Autodesk Inventor part; units mm, degrees
ref_plane "Work Plane1" through (-6.65, 6.65, 6.5) normal (0, 1, 0) x (1, 0, 0)
ref_plane "YZ Plane" through (0, 0, 0) normal (1, 0, 0) x (0, 1, 0)
ref_plane "XZ Plane" through (0, 0, 0) normal (0, 1, 0) x (-1, 0, 0)
sketch "Sketch1" plane through (0, 0, 0) normal (0, 0, 1) x (1, 0, 0)
  circle A0 centre (0, 0) radius 6.65
  dimension "d0" = 13.3
extrude "Extrusion1" add sketch "Sketch1" along normal blind 6.5
ref_plane "Work Plane1" through (-6.65, 6.65, 6.5) normal (0, 1, 0) x (1, 0, 0)
sketch "Sketch3" plane through (-6.65, 6.65, 6.5) normal (0, 1, 0) x (1, 0, 0)
  circle A0 centre (6.65, 3.25) radius 1.2
  dimension "d9" = 2.4
hole "Hole1" at (0, 6.65, 3.25) direction (0, -1, 0) diameter 2.459 depth 6.65
sketch "Sketch4" plane through (0, 0, 6.5) normal (0, 0, 1) x (1, 0, 0)
  circle A0 centre (0, 0) radius 6.65
  circle A1 centre (0, 0) radius 3
  dimension "d17" = 6
extrude "Extrusion3" add sketch "Sketch4" along normal blind 4.7 contours A1
properties part number "hridel kuzelova kolecka"
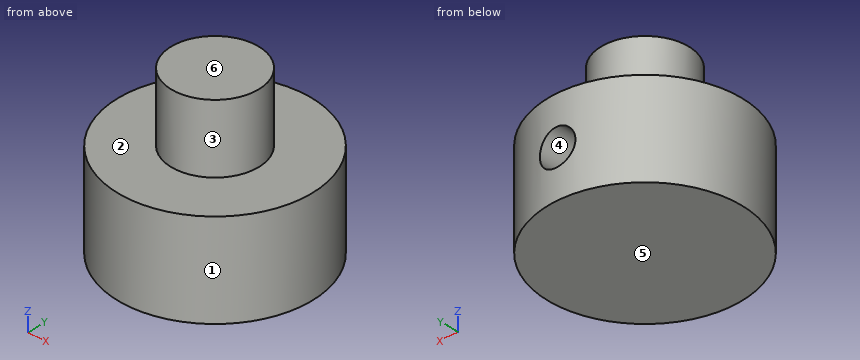
The model under review builds one solid part; all positions refer to its coordinate system, in mm. Face numbers are marked on the shaded views. A direction names the side the tool comes from. Give positions to 0.01 mm unless a question says otherwise; leave off trailing zeros. Write each loop counter-clockwise with the first axis right and the second up, starting at its lowest first coordinate (ties: lowest second). Pieces come first, ordered by that corner, then holes. Notation, with made-up numbers: M 10,68.5 L 50,68.5 A22 cw 50,104.5 Z; hole C 83,-18.5 d9. An arc over 180 degrees is marked long. Write item = value, one per line. Start each with the question number.
Q1. We need section A-A (y = 0.25). State the section outline as (x, z) points, plus the area to 3 significant figures.
Q2. We need section D-D (z = 7.25). State the section outline as (x, y) points, plus the area to 3 significant figures.
Q3. We need section C-C (y = -1.5). State the section outline as (x, z) points, plus the area to 3 significant figures.
Q4. Clearance check with flat-ended pins moving along their axes: pin 1 (1 mm diameter, centred on y = -1.5, z = 8.5, fed in from -X); pin 2 (2 mm diameter, centred on x = -2, z = 9.5, fed in from +Y); pin 3 (4 mm diameter, centred on x = 4.5, y = 3.5, fed in from +Z). State where each tip first meets the part, or that it passes through.
Q5. Mouldability with a two-part tool opening along Z and no side actions: class the marked faces 3, 4, 5 and 6 as released by +Z, released by -Z, zero draft, split by the parting line, or undercut.
Q6. Machinability: for the marked faces 1 and 2, which of the approach directions +Z, -Z, +X, -X, +Y, -Y give a long, thin tool a straight path to every point of the face, cutting with its end or side? Answer none if there is none.
Q7. We need section B-B (x = 0). State the section outline as (y, z) points, plus the area to 3 significant figures.
Q8. For line 1 (Z direction, x = 0, y = 5.75); line 2 (Z direction, x = 0, y = 2.5); line 3 (Z direction, x = 1.25, y = -3.5), list the stretches that pass through material, from the lowest coordinate up.
Result set:
q1.outline = M -6.65,0 L 6.65,0 L 6.65,6.5 L 2.99,6.5 L 2.99,11.2 L -2.99,11.2 L -2.99,6.5 L -6.65,6.5 Z; hole C 0,3.25 d2.46
q1.area = 110 mm2
q2.outline = C 0,0 d6
q2.area = 28.3 mm2
q3.outline = M -6.48,0 L 6.48,0 L 6.48,6.5 L 2.6,6.5 L 2.6,11.2 L -2.6,11.2 L -2.6,6.5 L -6.48,6.5 Z
q3.area = 109 mm2
q4.pin_1 = -2.83
q4.pin_2 = 2.83
q4.pin_3 = 6.5
q5.face_3 = zero draft
q5.face_4 = undercut
q5.face_5 = released by -Z
q5.face_6 = released by +Z
q6.face_1 = +Z, -Z
q6.face_2 = +Z
q7.outline = M -6.65,0 L 6.65,0 L 6.65,2.02 L 0,2.02 L 0,4.48 L 6.65,4.48 L 6.65,6.5 L 3,6.5 L 3,11.2 L -3,11.2 L -3,6.5 L -6.65,6.5 Z
q7.area = 98.3 mm2
q8.line_1 = 0 to 2.02, 4.48 to 6.5
q8.line_2 = 0 to 2.02, 4.48 to 11.2
q8.line_3 = 0 to 6.5
